from build123d import *

# Parameters (mm, degrees)
ESQUISSE1_R        = 1.1
BOSS_EXTRU_1_DEPTH = 0.8


with BuildPart() as part:
    # Esquisse1 → Boss.-Extru.1 (new body, symmetric)
    with BuildSketch(Plane(origin=(0, 0, 0), x_dir=(1, 0, 0), z_dir=(0, 1, 0))):
        with BuildLine():
            ThreePointArc((-12, -10), (-10, -12), (-8, -10))
            Line((-8, -10), (7.9, -10))
            ThreePointArc((7.9, -10), (10, -7.9), (12.1, -10))
            Line((12.1, -10), (19.2, -10))
            ThreePointArc((19.2, -10), (19.765685425, -9.765685425), (20, -9.2))
            Line((20, -9.2), (20, -2))
            ThreePointArc((20, -2), (22, 0), (20, 2))
            Line((20, 2), (20, 9.2))
            ThreePointArc((20, 9.2), (19.765685425, 9.765685425), (19.2, 10))
            Line((19.2, 10), (12.1, 10))
            ThreePointArc((12.1, 10), (10, 7.9), (7.9, 10))
            Line((7.9, 10), (-8, 10))
            ThreePointArc((-8, 10), (-10, 12), (-12, 10))
            Line((-12, 10), (-19.2, 10))
            ThreePointArc((-19.2, 10), (-19.765685425, 9.765685425), (-20, 9.2))
            Line((-20, 9.2), (-20, 2.1))
            ThreePointArc((-20, 2.1), (-17.9, 0), (-20, -2.1))
            Line((-20, -2.1), (-20, -9.2))
            ThreePointArc((-20, -9.2), (-19.765685425, -9.765685425), (-19.2, -10))
            Line((-19.2, -10), (-12, -10))
        make_face()
        with Locations((-10, -10)):
            Circle(ESQUISSE1_R, mode=Mode.SUBTRACT)
        with Locations((20, 0)):
            Circle(ESQUISSE1_R, mode=Mode.SUBTRACT)
        with Locations((-10, 10)):
            Circle(ESQUISSE1_R, mode=Mode.SUBTRACT)
    extrude(amount=BOSS_EXTRU_1_DEPTH, both=True)


solid = part.part
Design review of the part built by this model. Coordinates are the model's own, in mm. A direction names the side the tool comes from. Give positions to 0.01 mm unless a question says otherwise; leave off trailing zeros. Loops run counter-clockwise (first coordinate to the right, second up) from the corner with the lowest first, then second, coordinate; pieces in that order, holes last. Notation, with made-up numbers: (31.25, -26) - (52.25, -26) arc R22 cw to (52.25, 13) - close; hole circle Ø10 at (34, 61.25). An arc over 180 degrees is marked (long way). Write item = value, one per line.
1) Take a section at B-B on y = 0. State the section outline as (x, z) points.
Result sheet:
outline = (-20, -9.2) arc R0.8 ccw to (-19.2, -10) - (-12, -10) arc R2 ccw to (-8, -10) - (7.9, -10) arc R2.1 cw to (12.1, -10) - (19.2, -10) arc R0.8 ccw to (20, -9.2) - (20, -2) arc R2 ccw to (20, 2) - (20, 9.2) arc R0.8 ccw to (19.2, 10) - (12.1, 10) arc R2.1 cw to (7.9, 10) - (-8, 10) arc R2 ccw to (-12, 10) - (-19.2, 10) arc R0.8 ccw to (-20, 9.2) - (-20, 2.1) arc R2.1 cw to (-20, -2.1) - close; hole circle Ø2.2 at (-10, -10); hole circle Ø2.2 at (-10, 10); hole circle Ø2.2 at (20, 0)
2) Take a section at D-D on z = -3. State the section outline as (x, y) points.
Result sheet:
outline = (-20, -0.8) - (20, -0.8) - (20, 0.8) - (-20, 0.8) - close
3) Take a section at C-C on x = -14. State the section outline as (y, z) points.
Result sheet:
outline = (-0.8, -10) - (0.8, -10) - (0.8, 10) - (-0.8, 10) - close
4) Draft analysis for pull direction X (two halves, no side actions). For faces 5 (the face through (-10, 0, 12)), 6 (the face through (10, 0, -7.9)), 7 (the face through (0, 0, 10)), state which applies: +X half, -X half, draft (parallel to the pull), parting line (faces both ways), or undercut.
Result sheet:
face_5 = parting line
face_6 = undercut
face_7 = draft
5) Tool access review of faces 1 (the face through (20, 0, -6)), 2 (the face through (16, 0, 10)), 3 (the face through (-16, 0, -10)), 4 (the face through (1, -0.8, 0)): name each direction out of +Z, -Z, +X, -X, +Y, -Y from which nothing blocks a thin tool from reaching the whole face with its end or side.
Result sheet:
face_1 = -Z, +X, +Y, -Y
face_2 = +Z, +X, +Y, -Y
face_3 = -Z, -X, +Y, -Y
face_4 = +Z, -Z, +X, -X, -Y
6) Clearance check with flat-ended pins moving along their axes: pin 1 Ø0.5 at (x, y) = (-15, 0) entering from -Z; pin 2 Ø0.5 at (y, z) = (0, 4.5) entering from +X; pin 3 Ø3.5 at (x, z) = (-10, 10) entering from +Y; pin 4 Ø1.3 at (x, z) = (-10, -10) entering from +Y. State where each tip first meets the part, or that it passes through.
Result sheet:
pin_1 = -10
pin_2 = 20
pin_3 = 0.8
pin_4 = through
7) To check wall thickness, follow line 1 (Z direction, x = -10, y = 0.45); line 2 (X direction, y = -0.55, z = -9.25); line 3 (X direction, y = 0.25, z = 0). State the ranges of each line that lie inside material, in increasing order.
Result sheet:
line_1 = -12 to -11.1, -8.9 to 8.9, 11.1 to 12
line_2 = -20 to -10.8, -9.2 to 8.04, 11.96 to 20
line_3 = -17.9 to 18.9, 21.1 to 22
8) Take a section at A-A on z = 0. State the section outline as (x, y) points.
Result sheet:
outline = (-17.9, -0.8) - (18.9, -0.8) - (18.9, 0.8) - (-17.9, 0.8) - close; (21.1, -0.8) - (22, -0.8) - (22, 0.8) - (21.1, 0.8) - close
